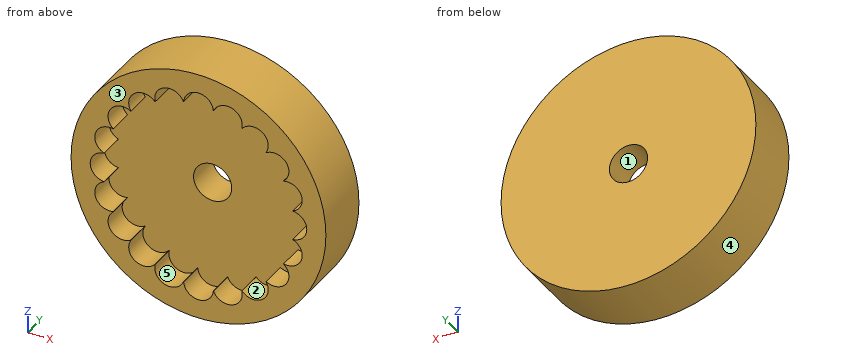
```python
from build123d import *

# Parameters (mm, degrees)
CYLINDER043_R           = 15
CYLINDER043_DEPTH       = 7
CYLINDER044_R           = 11.25
CYLINDER044_DEPTH       = 3
CYLINDER045_R           = 1.75
CYLINDER045_DEPTH       = 3
POLARPATTERN009_COUNT   = 20
CYLINDER048_R           = 2.25
CYLINDER048_DEPTH       = 7
BODY019_PLACEMENT_ANGLE = 90


with BuildPart() as part:
    # Cylinder043 → Cylinder043 (join)
    with BuildSketch(Plane(origin=(0, 0, 3), x_dir=(-1, 0, 0), z_dir=(0, 0, -1))):
        Circle(CYLINDER043_R)
    extrude(amount=CYLINDER043_DEPTH)

    # Cylinder044 → Cylinder044 (cut)
    with BuildSketch(Plane.XY):
        Circle(CYLINDER044_R)
    extrude(amount=CYLINDER044_DEPTH, mode=Mode.SUBTRACT)

    # Cylinder045 → Cylinder045 (cut)
    with BuildSketch(Plane(origin=(0, 11, 0), x_dir=(1, 0, 0), z_dir=(0, 0, 1))):
        Circle(CYLINDER045_R)
    cylinder045 = extrude(amount=CYLINDER045_DEPTH, mode=Mode.SUBTRACT)

    # PolarPattern009: Cylinder045 ×20 about axis
    polarpattern009_axis = Axis((0, 0, 0), (0, 0, 1))
    for i in range(1, POLARPATTERN009_COUNT):
        add(cylinder045.rotate(polarpattern009_axis, i * 360 / POLARPATTERN009_COUNT), mode=Mode.SUBTRACT)

    # Cylinder048 → Cylinder048 (cut)
    with BuildSketch(Plane.XY.offset(-7)):
        Circle(CYLINDER048_R)
    extrude(amount=CYLINDER048_DEPTH, mode=Mode.SUBTRACT)


with BuildPart() as part_1:
    # Body019 placement: moved
    add(part.part.moved(Location((0, 7, 60))).rotate(Axis((0, 7, 60), (1, 0, 0)), BODY019_PLACEMENT_ANGLE))


solid = part_1.part
```
Verification items for the finished model (mm, model axes). Face numbers are marked on the shaded views. A direction names the side the tool comes from. Coordinates: 2 decimals unless noted, no trailing zeros. Write each loop counter-clockwise with the first axis right and the second up, starting at its lowest first coordinate (ties: lowest second). Pieces come first, ordered by that corner, then holes. Notation, with made-up numbers: (9, 20.5) - (13, 20.5) arc R12 ccw to (13, 27.5) - close; hole circle Ø3 at (52.25, 45.25). An arc over 180 degrees is marked (long way). Write item = value, one per line.
Q1. Mould release check, pull along Z, two halves, no side actions. Record for the marked faces 3, 4 and 5: released by +Z, released by -Z, zero draft, split by the parting line, or undercut.
Answer:
face_3 = zero draft
face_4 = split by the parting line
face_5 = undercut
Q2. Cross-section at D-D (x = 4.25). Enter the section's corners in (y, z), plus the area to 3 significant figures.
Answer:
outline = (4, 45.61) - (11, 45.61) - (11, 74.39) - (4, 74.39) - (4, 71.99) - (7, 71.99) - (7, 48.01) - (4, 48.01) - close
area = 129 mm²
Q3. Material ranges on L1, parallel to Z at x = 0, y = 9.05; L2, parallel to Z at x = 12, y = 5.5; L3, parallel to Y at x = 10.5, z = 67, recorded low to high. Write a range as from..to.
Answer:
L1 = 45..57.75, 62.25..75
L2 = 51..55.77, 57.44..58.56, 61.44..62.56, 64.23..69
L3 = 7..11
Q4. Go/stop test with flat-tipped pins: pin 1 Ø7.5 at (x, z) = (-0.5, 58) entering from -Y; pin 2 Ø1 at (y, z) = (10, 68) entering from -X; pin 3 Ø2.5 at (x, z) = (0, 60) entering from -Y; pin 4 Ø4 at (y, z) = (7.5, 71.5) entering from +X. Record where each tip stops, or that it passes through.
Answer:
pin_1 = 7
pin_2 = -12.99
pin_3 = through
pin_4 = 11.61
Q5. Cross-section at B-B (z = 60). Enter the section's corners in (x, y), plus the area to 4 significant figures.
Answer:
outline = (-15, 4) - (-12.75, 4) - (-12.75, 7) - (-2.25, 7) - (-2.25, 11) - (-15, 11) - close; (2.25, 7) - (12.75, 7) - (12.75, 4) - (15, 4) - (15, 11) - (2.25, 11) - close
area = 115.5 mm²
Q6. Cross-section at C-C (y = 9.5). Enter the section's corners in (x, z), plus the area to 3 significant figures.
Answer:
outline = circle Ø30 at (0, 60); hole circle Ø4.5 at (0, 60)
area = 691 mm²
Q7. Access from +Z, -Z, +X, -X, +Y, -Y to the whole of each face (thin tool, end or side, straight path). Record for the marked faces 1 and 2.
Answer:
face_1 = +Y, -Y
face_2 = -Y
Q8. Cross-section at A-A (x = 0). Enter the section's corners in (y, z).
Answer:
outline = (4, 45) - (11, 45) - (11, 57.75) - (7, 57.75) - (7, 47.25) - (4, 47.25) - close; (4, 72.75) - (7, 72.75) - (7, 62.25) - (11, 62.25) - (11, 75) - (4, 75) - close
